Input: part model. Units: mm. Frame: model coordinates. A direction names the side the tool comes from. Round coordinates to 2 decimals unless told otherwise and drop trailing zeros. Loops run counter-clockwise (first coordinate to the right, second up) from the corner with the lowest first, then second, coordinate; pieces in that order, holes last. Notation, with made-up numbers: (7.25, 60.25) -> (26.25, 60.25) arc R15 cw to (26.25, 72.25) -> close; hole circle Ø8 at (51, 60). An arc over 180 degrees is marked (long way). Answer in a Markdown table with one row per item. Add a question column.
Q1. Mould query, pull axis X, two halves, no side actions, for faces 1 (the face through (-4, -6, 8)), 2 (the face through (6.816, 12.067, 3.944)), 3 (the face through (2.88, -6.06, 3.94)). Classes: pulls with the +X half, pulls with the -X half, needs draft (parallel to the pull), parting line crosses it, or undercut.
Q2. Reachability of faces 4 (the face through (-4.87, -4.614, 3.944)), 5 (the face through (-3.713, 13.352, 3.944)) from +Z, -Z, +X, -X, +Y, -Y: full face, straight path, thin tool, end or side. Return the list, or none.
Q3. Pin query (flat end, axial travel): pin 1 (1 mm diameter, centred on x = 8.5, y = -3, fed in from -Z); pin 2 (2 mm diameter, centred on x = 7, z = 1, fed in from -Y); pin 3 (4 mm diameter, centred on y = 4, z = 7, fed in from +X); pin 4 (4 mm diameter, centred on x = -9.5, z = 1.5, fed in from +Y). Return the tip coordinate at first contact, or that it passes through.
Q4. Ray query, L1, parallel to Y at x = 2, z = 3.75; L2, parallel to X at y = -2.75, z = 7.25; L3, parallel to Y at x = -0.5, z = 3.5. Return the intervals inside material, ascending. Write a range as from..to.
Q5. Section A-A, the plane y = -2.5. Output: boundary loops of the cut face in (x, z), and give its area (3 significant figures).
Q6. Section B-B, the plane z = 1. Output: boundary loops of the cut face in (x, y).
Q7. Section D-D, the plane y = 10. Output: boundary loops of the cut face in (x, z), and give its area (3 significant figures).
Q8. Section C-C, the plane x = -4.5. Output: boundary loops of the cut face in (y, z), and give its area (3 significant figures).
```python
from build123d import *

# Parameters (mm, degrees)
F1_DEPTH = 8


with BuildPart() as f1:
    # F0 (on Top) → F1 (new body)
    with BuildSketch(Plane.XY):
        Polygon((-9.311619, 11.759837), (-14.899769, 1.731152), (-11.759837, -9.311619), (-1.731152, -14.899769), (9.311619, -11.759837), (14.899769, -1.731152), (11.759837, 9.311619), (1.731152, 14.899769), align=None)
        Polygon((-1.600227, -8.135918), (-8.232215, -0.992231), (-3.487562, 7.522685), (6.076783, 5.641506), (7.24322, -4.036043), align=None, mode=Mode.SUBTRACT)
    extrude(amount=F1_DEPTH)


solid = f1.part
```
Answer block:
| question | item | result |
|---|---|---|
| 1 | face 1 | needs draft |
| 1 | face 2 | pulls with the +X half |
| 1 | face 3 | undercut |
| 2 | face 4 | +Z, -Z |
| 2 | face 5 | +Z, -Z, -X, +Y |
| 3 | pin 1 | z = 0 |
| 3 | pin 2 | y = -12.7 |
| 3 | pin 3 | x = 13.84 |
| 3 | pin 4 | y = 12.27 |
| 4 | L1 | -13.84..-6.47, 6.44..14.75 |
| 4 | L2 | -13.63..-6.6, 7.09..14.33 |
| 4 | L3 | -14.55..-7.63, 6.94..14.27 |
| 5 | outline | (-13.7, 0) -> (-6.83, 0) -> (-6.83, 8) -> (-13.7, 8) -> close; (7.06, 0) -> (14.47, 0) -> (14.47, 8) -> (7.06, 8) -> close |
| 5 | area | 114 mm^2 |
| 6 | outline | (-14.9, 1.73) -> (-11.76, -9.31) -> (-1.73, -14.9) -> (9.31, -11.76) -> (14.9, -1.73) -> (11.76, 9.31) -> (1.73, 14.9) -> (-9.31, 11.76) -> close; hole (-8.23, -0.99) -> (-1.6, -8.14) -> (7.24, -4.04) -> (6.08, 5.64) -> (-3.49, 7.52) -> close |
| 7 | outline | (-10.29, 0) -> (10.52, 0) -> (10.52, 8) -> (-10.29, 8) -> close |
| 7 | area | 167 mm^2 |
| 8 | outline | (-13.36, 0) -> (-5.01, 0) -> (-5.01, 8) -> (-13.36, 8) -> close; (5.71, 0) -> (13.13, 0) -> (13.13, 8) -> (5.71, 8) -> close |
| 8 | area | 126 mm^2 |
